Verification items for this drawing (mm, ordinates from the low corner). A direction names the side the tool comes from. Coordinates: 2 decimals unless noted, no trailing zeros. Write each loop counter-clockwise with the first axis right and the second up, starting at its lowest first coordinate (ties: lowest second). Pieces come first, ordered by that corner, then holes. Notation, with made-up numbers: M -24.5,13 L 19.5,13 A31 cw 19.5,51 Z; hole C 28.25,35.5 d6. An arc over 180 degrees is marked long. Write each question's results on one line, items separated by ' | '.
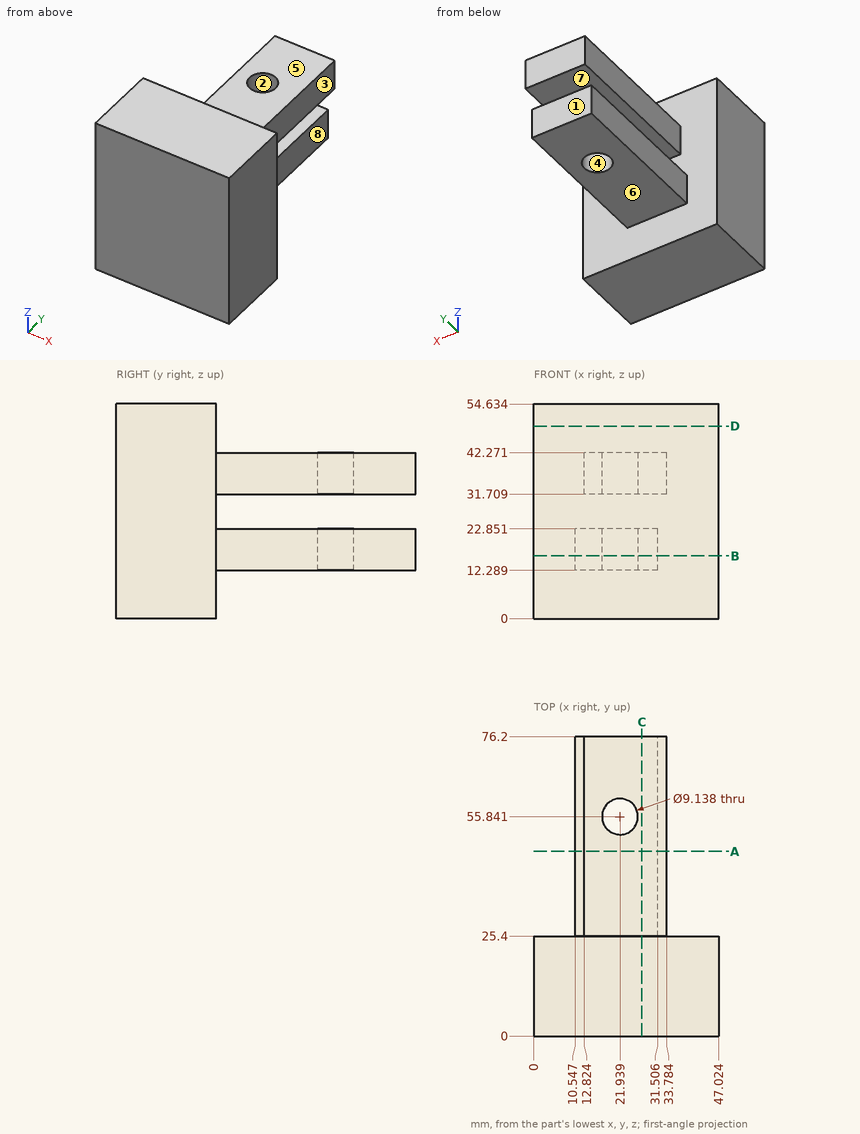
Q1. Sectioned sample at C-C on x = 27.5. Record the cut outline in (y, z) (1 decimal).
Geometry check:
outline: M 0,0 L 25.4,0 L 25.4,12.3 L 76.2,12.3 L 76.2,22.9 L 25.4,22.9 L 25.4,31.7 L 76.2,31.7 L 76.2,42.3 L 25.4,42.3 L 25.4,54.6 L 0,54.6 Z
Q2. Sectioned sample at A-A on y = 47. Record the cut outline in (x, z).
Geometry check:
outline: M 10.55,12.29 L 31.51,12.29 L 31.51,22.85 L 10.55,22.85 Z; M 12.82,31.71 L 33.78,31.71 L 33.78,42.27 L 12.82,42.27 Z
Q3. Access from +Z, -Z, +X, -X, +Y, -Y to the whole of each face (thin tool, end or side, straight path). Record for the marked faces 5, 6, 7 and 8.
Geometry check:
face 5: +Z, +X, -X, +Y | face 6: -Z, +X, -X, +Y | face 7: +X, -X, +Y | face 8: -Z, +X, +Y
Q4. Scan lines: probe 1 along Z at (x, y) = (28.5, 39); probe 2 along Y at (x, z) = (41, 2.5); probe 3 along Z at (x, y) = (33.5, 51.5). Record each from-to range of solid material in increasing order.
Geometry check:
probe 1: z = 12.29 to 22.85, 31.71 to 42.27 | probe 2: y = 0 to 25.4 | probe 3: z = 31.71 to 42.27
Q5. Sectioned sample at D-D on z = 49. Record the cut outline in (x, y) (1 decimal).
Geometry check:
outline: M 0,0 L 47,0 L 47,25.4 L 0,25.4 Z
Q6. Sectioned sample at B-B on z = 16. Record the cut outline in (x, y) (1 decimal), and give its area (3 significant figures).
Geometry check:
outline: M 0,0 L 47,0 L 47,25.4 L 31.5,25.4 L 31.5,76.2 L 10.5,76.2 L 10.5,25.4 L 0,25.4 Z; hole C 21.9,55.8 d9.1 | area: 2,190 mm2
Q7. Depth check by flat-ended pin: P1, Ø8.5, axis at y = 56, z = 19.5, coming from the -X side; P2, Ø3, axis at y = 60, z = 20, coming from the +X side; P3, Ø6.5, axis at x = 25.5, y = 42.5, coming from the +Z side. Enter the tip coordinate at first touch or a pass-through.
Geometry check:
P1: stops at x = 10.55 | P2: stops at x = 31.51 | P3: stops at z = 42.27
Q8. Mould release check, pull along X, two halves, no side actions. Record for the marked faces 1, 2, 3 and 4: pulls with the +X half, pulls with the -X half, needs draft (parallel to the pull), parting line crosses it, or undercut.
Geometry check:
face 1: needs draft | face 2: undercut | face 3: pulls with the +X half | face 4: undercut
